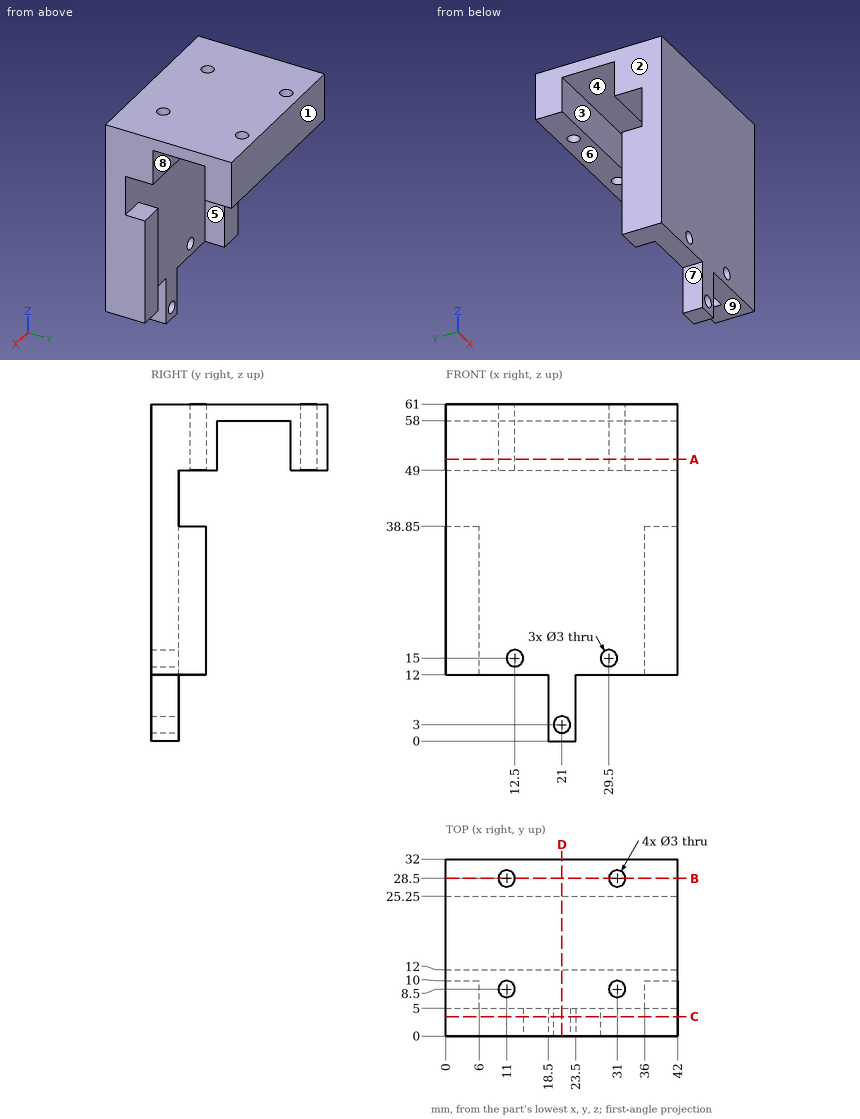
Geometry: see drawing. Coordinates: mm, zero at the bounding-box minimum. A direction names the side the tool comes from. Round coordinates to 2 decimals unless told otherwise and drop trailing zeros. Order: outer loops, then holes, each group sorted by start corner. A loop starts at its lowest first (then second) coordinate and runs counter-clockwise, first axis right, second up. Notation, with made-up numbers: (40, -6) - (80, -6) arc R15 cw to (80, -2) - close; hole circle Ø10 at (-0.5, -40). An arc over 180 degrees is marked (long way). One line per question, with ' | ' between items. Start each with the question number.
1) Cut plane A-A, the plane z = 51. Return the cut outline in (x, y).
2) Cut plane D-D, the plane x = 21. Return the cut outline in (y, z), then the cut area to 3 significant figures.
3) Ray query, probe 1 along Y at (x, z) = (31, 53); probe 2 along X at (y, z) = (5.5, 25); probe 3 along Y at (x, z) = (2.5, 55.5). Return the intervals inside material, ascending.
4) Contact query for flat-ended pins moving along their axis: P1, Ø1, axis at x = 19.5, z = 13.5, coming from the +Y side; P2, Ø5, axis at x = 11, y = 28.5, coming from the +Z side; P3, Ø4, axis at y = 3.5, z = 4.5, coming from the -X side; P4, Ø14.5, axis at x = 21, y = 17.5, coming from the -Z side. Output: stop coordinate, or through.
5) Cut plane B-B, the plane y = 28.5. Return the cut outline in (x, z).
6) Set-up query: the marked faces 5, 6, 7, 8 and 9. Return all of +Z, -Z, +X, -X, +Y, -Y with unobstructed straight access to the full face (end or side cutting, diameter ignored); none if empty.
7) Cut plane C-C, the plane y = 3.5. Return the cut outline in (x, z).
8) Pull-direction query (Y, two-part tool) for the marked faces 1, 2, 3 and 4; classes: +Y half, -Y half, draft (parallel to the pull), parting line (faces both ways), or undercut.
Worked out:
1) outline: (0, 0) - (42, 0) - (42, 12) - (0, 12) - close; (0, 25.25) - (42, 25.25) - (42, 32) - (0, 32) - close; hole circle Ø3 at (11, 8.5); hole circle Ø3 at (11, 28.5); hole circle Ø3 at (31, 8.5); hole circle Ø3 at (31, 28.5)
2) outline: (0, 0) - (5, 0) - (5, 1.5) - (0, 1.5) - close; (0, 4.5) - (5, 4.5) - (5, 49) - (12, 49) - (12, 58) - (25.25, 58) - (25.25, 49) - (32, 49) - (32, 61) - (0, 61) - close | area: 495 mm^2
3) probe 1: y = 0 to 7, 10 to 12, 25.25 to 27, 30 to 32 | probe 2: x = 0 to 6, 36 to 42 | probe 3: y = 0 to 12, 25.25 to 32
4) P1: stops at y = 5 | P2: stops at z = 61 | P3: stops at x = 18.5 | P4: stops at z = 49
5) outline: (0, 49) - (9.5, 49) - (9.5, 61) - (0, 61) - close; (12.5, 49) - (29.5, 49) - (29.5, 61) - (12.5, 61) - close; (32.5, 49) - (42, 49) - (42, 61) - (32.5, 61) - close
6) face 5: -Z, +Y | face 6: -Z, +X, -X, +Y | face 7: -Z, -X, +Y, -Y | face 8: -Z, +X, -X | face 9: -Z, +X, +Y, -Y
7) outline: (0, 12) - (18.5, 12) - (18.5, 0) - (23.5, 0) - (23.5, 12) - (42, 12) - (42, 61) - (0, 61) - close; hole circle Ø3 at (12.5, 15); hole circle Ø3 at (21, 3); hole circle Ø3 at (29.5, 15)
8) face 1: +Y half | face 2: draft | face 3: undercut | face 4: undercut
